Read the model definition and answer for the solid it produces. Units are mm, in the model's axes. Round coordinates to 2 decimals unless told otherwise and drop trailing zeros. Loops run counter-clockwise (first coordinate to the right, second up) from the corner with the lowest first, then second, coordinate; pieces in that order, holes last. Notation, with made-up numbers: (-34.5, 53.5) - (10.5, 53.5) arc R24 ccw to (10.5, 84.5) - close; hole circle Ø6 at (27, 78). An arc over 180 degrees is marked (long way). Answer as CSV lines item,"result".
```python
from build123d import *


with BuildPart() as part:
    # Эскиз1 → Повернуть-Тонкостенный3 (revolve)
    with BuildSketch(Plane(origin=(0, 0, 0), x_dir=(0, 0, -1), z_dir=(1, 0, 0))):
        with BuildLine():
            ThreePointArc((1, 0), (105.7166575, 16.855175566), (200, 65.438368426))
            Line((200, 65.438368426), (200, 934.561631574))
            ThreePointArc((200, 934.561631574), (105.7166575, 983.144824434), (1, 1000))
            Line((1, 1000), (1.004453384, 1002.999996695))
            ThreePointArc((1.004453384, 1002.999996695), (107.375751508, 985.756396385), (203, 936.075435077))
            Line((203, 936.075435077), (203, 63.924564923))
            ThreePointArc((203, 63.924564923), (107.375751508, 14.243603615), (1.004453384, -2.999996695))
            Line((1.004453384, -2.999996695), (1, 0))
        make_face()
    revolve(axis=Axis((0, -42.73513709, 0), (0, 1, 0)))


solid = part.part
```
1) A cutting plane is placed at A-A, the plane y = 380.5. Determine the outline of the cut face in (x, z), plus the area to 3 significant figures.
Entries:
outline,"circle Ø406 at (0, 0); hole circle Ø400 at (0, 0)"
area,"3,800 mm^2"
2) Each of these flat-tipped pins is pushed along its axis until it touches: P1, Ø1, axis at x = 22, z = 121, coming from the +Y side; P2, Ø3, axis at y = 794.5, z = 58.5, coming from the -X side; P3, Ø1, axis at x = -107, y = 406.5, coming from the -Z side. Where does it stop, or does it pass through?
Entries:
P1,"stops at y = 980.35"
P2,"stops at x = -194.83"
P3,"stops at z = -172.82"
3) Find the intervals of material crossed by line 1 (X direction, y = 466, z = 0); line 2 (X direction, y = 464.5, z = -5), in increasing order.
Entries:
line 1,"x = -203 to -200, 200 to 203"
line 2,"x = -202.94 to -199.94, 199.94 to 202.94"
4) The mould has two halves that part along Z. Classify faces 1 (the face through (-60.976, 493.895, -193.626)), 2 (the face through (-60.075, 506.084, -190.764)): pulls with the +Z half, pulls with the -Z half, needs draft (parallel to the pull), parting line crosses it, or undercut.
Entries:
face 1,"parting line crosses it"
face 2,"undercut"
